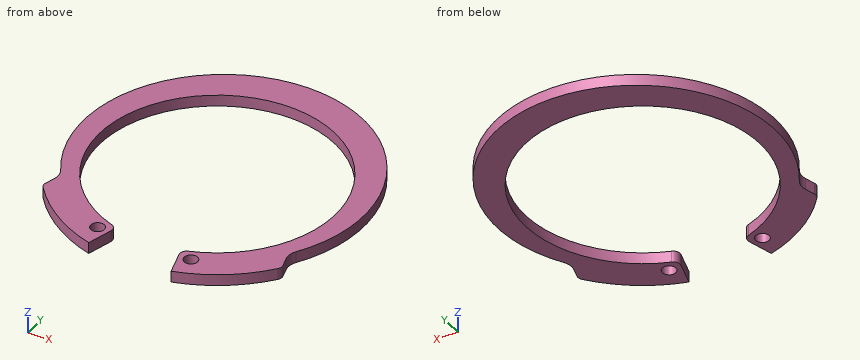
from build123d import *

# Parameters (mm, degrees)
BODYSKE_R  = 0.381
BODY_DEPTH = 0.635


with BuildPart() as part:
    # BodySke → Body (new body)
    with BuildSketch(Plane.XY):
        with BuildLine():
            Line((-1.91450535, -6.719919163), (-2.314042344, -8.122295136))
            ThreePointArc((-2.314042344, -8.122295136), (-4.67753589, -7.031865204), (-6.59672094, -5.273494391))
            ThreePointArc((-6.59672094, -5.273494391), (-6.672649179, -5.110694444), (-6.665543836, -4.931199501))
            Line((-6.665543836, -4.931199501), (-6.501980098, -4.357090321))
            ThreePointArc((-6.501980098, -4.357090321), (-6.476670268, -3.974948798), (-6.610396151, -3.616075396))
            ThreePointArc((-6.610396151, -3.616075396), (0, 8.4455), (6.610396151, -3.616075396))
            ThreePointArc((6.610396151, -3.616075396), (6.476670268, -3.974948798), (6.501980098, -4.357090321))
            Line((6.501980098, -4.357090321), (6.665543836, -4.931199501))
            ThreePointArc((6.665543836, -4.931199501), (6.672649179, -5.110694444), (6.59672094, -5.273494391))
            ThreePointArc((6.59672094, -5.273494391), (4.67753589, -7.031865204), (2.314042344, -8.122295136))
            Line((2.314042344, -8.122295136), (1.91450535, -6.719919163))
            ThreePointArc((1.91450535, -6.719919163), (1.943087835, -6.439380692), (2.156736403, -6.255334282))
            ThreePointArc((2.156736403, -6.255334282), (0, 6.6167), (-2.156736403, -6.255334282))
            ThreePointArc((-2.156736403, -6.255334282), (-1.943087835, -6.439380692), (-1.91450535, -6.719919163))
        make_face()
        with Locations((2.620803478, -6.78878292)):
            Circle(BODYSKE_R, mode=Mode.SUBTRACT)
        with Locations((-2.620803478, -6.78878292)):
            Circle(BODYSKE_R, mode=Mode.SUBTRACT)
    extrude(amount=-BODY_DEPTH)


solid = part.part
Work out the finished part from the listing and answer in its coordinate system (mm). Give positions to 0.01 mm unless a question says otherwise; leave off trailing zeros. Write each loop counter-clockwise with the first axis right and the second up, starting at its lowest first coordinate (ties: lowest second). Pieces come first, ordered by that corner, then holes. Notation, with made-up numbers: M -22,36.25 L 8,36.25 A23 cw 8,55.25 Z; hole C 27.25,23 d11. An arc over 180 degrees is marked long. Answer as CSV lines item,"result".
Q1. Find the intervals of material crossed by probe 1 along X at (y, z) = (0.5, -0.1); probe 2 along X at (y, z) = (-4.5, -0.25); probe 3 along Y at (x, z) = (3.5, -0.55), in increasing order. Write a range as [from, to].
A:
probe 1,"x = [-7.84, -6.6], [6.6, 7.84]"
probe 2,"x = [-6.54, -4.85], [4.85, 6.54]"
probe 3,"y = [-7.69, -5.62], [5.62, 7.62]"
Q2. A cutting plane is placed at D-D on x = -5.5. Write down the section's boundary in (y, z) (3 decimals), plus the area to 3 significant figures.
A:
outline,"M -6.409,-0.635 L -3.678,-0.635 L -3.678,0 L -6.409,0 Z; M 3.678,-0.635 L 6.193,-0.635 L 6.193,0 L 3.678,0 Z"
area,"3.33 mm²"
Q3. A cutting plane is placed at C-C on x = 2.75. Write down the section's boundary in (y, z) (3 decimals), plus the area to 3 significant figures.
A:
outline,"M -7.985,-0.635 L -7.147,-0.635 L -7.147,0 L -7.985,0 Z; M -6.43,-0.635 L -6.018,-0.635 L -6.018,0 L -6.43,0 Z; M 6.018,-0.635 L 7.948,-0.635 L 7.948,0 L 6.018,0 Z"
area,"2.02 mm²"
Q4. A cutting plane is placed at A-A on y = 0. Write down the section's boundary in (x, z) (3 decimals), plus the area to 3 significant figures.
A:
outline,"M -7.819,-0.635 L -6.617,-0.635 L -6.617,0 L -7.819,0 Z; M 6.617,-0.635 L 7.819,-0.635 L 7.819,0 L 6.617,0 Z"
area,"1.53 mm²"
Q5. A cutting plane is placed at B-B on z = -0.2. Write down the section's boundary in (x, y), plus the area to 3 significant figures.
A:
outline,"M -6.67,-4.93 A0.38 ccw -6.6,-5.27 A8.45 ccw -2.31,-8.12 L -1.91,-6.72 A0.38 ccw -2.16,-6.26 A6.62 cw long 2.16,-6.26 A0.38 ccw 1.91,-6.72 L 2.31,-8.12 A8.45 ccw 6.6,-5.27 A0.38 ccw 6.67,-4.93 L 6.5,-4.36 A0.91 cw 6.61,-3.62 A7.84 ccw long -6.61,-3.62 A0.91 cw -6.5,-4.36 Z; hole C -2.62,-6.79 d0.76; hole C 2.62,-6.79 d0.76"
area,"64.2 mm²"
